Autodesk Inventor part; units mm, degrees
ref_plane "Work Plane5" through (0, 0, 76.2) normal (0, 0, 1) x (1, 0, 0)
ref_plane "Work Plane6" through (0, 0, 15.113) normal (0, 0, -1) x (-1, 0, 0)
ref_plane "Work Plane10" through (0, 0, 29.464) normal (0, 0, -1) x (-1, 0, 0)
sketch "Sketch1" plane through (0, 0, 0) normal (0, 0, 1) x (1, 0, 0)
  circle A0 centre (0, 0) radius 12.7
  circle A1 centre (0, 0) radius 6.35
  line L0 (-1.5875, 14.2875) -> (1.5875, 14.2875)
  line L1 (1.5875, 14.2875) -> (1.5875, 11.1125)
  line L2 (1.5875, 11.1125) -> (-1.5875, 11.1125)
  line L3 (-1.5875, 11.1125) -> (-1.5875, 14.2875)
  dimension "d0" = 25.4
  dimension "d4" = 12.7
  dimension "d50" = 3.175
  dimension "d51" = 3.175
  dimension "d52" = 1.5875
  dimension "d53" = 14.2875
extrude "Extrusion4" add sketch "Sketch1" along normal blind 79.375 contours A0 L3 L2 L1 | L1 L2 L3 A0
ref_plane "Work Plane5" through (0, 0, 76.2) normal (0, 0, 1) x (1, 0, 0)
sketch "Sketch6" plane through (0, 0, 76.2) normal (0, 0, 1) x (1, 0, 0)
  circle A0 centre (0, 0) radius 12.192
  circle A1 centre (0, 0) radius 12.7
  dimension "d24" = 24.384
extrude "Extrusion8" cut sketch "Sketch6" along normal blind 1.143
ref_plane "Work Plane6" through (0, 0, 15.113) normal (0, 0, -1) x (-1, 0, 0)
ref_plane "Work Plane9" through (0, 0, 43.3324) normal (0, 0, -1) x (-1, 0, 0)
ref_plane "Work Plane10" through (0, 0, 29.464) normal (0, 0, -1) x (-1, 0, 0)
extrude "Extrusion16" cut sketch "Sketch1" along normal through all contours L1 L2 L3 A0 | A0 L3 L0 L1 picked at (0.1768, 11.638)
sketch "Sketch14" plane through (0, 0, 79.375) normal (0, 0, 1) x (1, 0, 0)
  circle A0 centre (0, 0) radius 6.35
  circle A1 centre (0, 0) radius 7.9375
  dimension "d56" = 15.875
extrude "Extrusion17" cut sketch "Sketch14" against normal blind 7.9375
sketch "Sketch15" plane through (0, 0, 0) normal (0, 0, -1) x (-1, 0, 0)
  circle A0 centre (0, 0) radius 6.35
  circle A1 centre (0, 0) radius 7.9375
  dimension "d59" = 15.875
extrude "Extrusion18" cut sketch "Sketch15" against normal blind 7.9375
ref_plane "Work Plane13" through (0, 0, 6.35) normal (0, 0, -1) x (-1, 0, 0)
sketch "Sketch16" plane through (0, 0, 6.35) normal (0, 0, -1) x (-1, 0, 0)
  arc A0 (-1.5875, 12.6004) -> (1.5875, 12.6004) centre (0, 0) ccw
  line L0 (-1.5875, 12.6004) -> (-1.5875, 11.1125)
  line L1 (-1.5875, 11.1125) -> (1.5875, 11.1125)
  line L2 (1.5875, 11.1125) -> (1.5875, 12.6004)
  circle A1 centre (0, 0) radius 15.875
  circle A2 centre (0, 0) radius 14.2875
  dimension "d63" = 31.75
  dimension "d68" = 28.575
extrude "Extrusion19" add sketch "Sketch16" against normal blind 3.175 contours A1 | A2
sketch "Sketch17" plane through (0, 0, 0) normal (0, 0, -1) x (-1, 0, 0)
  line L0 (-1.5875, 11.1125) -> (-1.5875, 12.6004)
  arc A0 (-1.5875, 12.6004) -> (1.5875, 12.6004) centre (0, 0) ccw
  line L1 (1.5875, 12.6004) -> (1.5875, 11.1125)
  line L2 (1.5875, 11.1125) -> (-1.5875, 11.1125)
  arc A1 (1.5875, 12.6004) -> (-1.5875, 12.6004) centre (0, 0) ccw
extrude "Extrusion20" add sketch "Sketch17" against normal blind 6.35 contours L0 A1 L1 L2
extrude "Extrusion21" add sketch "Sketch16" against normal blind 6.35 contours A2
equation "\"d51\" = d50"
properties part number "turn shaft 3"
For this review, take the finished solid that the model builds, in its own axes (mm). A direction names the side the tool comes from. Round coordinates to 2 decimals unless told otherwise and drop trailing zeros. Use CSV: the item, a comma, the result in double quotes.
1) Clearance check with flat-ended pins moving along their axes: pin 1 Ø1.6 at (x, z) = (-1, 51.5) entering from +Y; pin 2 Ø1.2 at (y, z) = (12, 48.5) entering from +X; pin 3 Ø2 at (x, z) = (-0.5, 40.5) entering from -Y; pin 4 Ø7.5 at (x, y) = (0, 0) entering from +Z. State where each tip first meets the part, or that it passes through.
Conclusion:
pin 1,"stops at y = 12.6"
pin 2,"stops at x = 5.6"
pin 3,"stops at y = -12.7"
pin 4,"passes through"
2) The part is to be moulded in two halves that separate along Z. For faces 1 (the flat face through (7, 11, 6.35)), 2 (the cylindrical face through (0.51, -12.18, 76.76)), 3 (the cylindrical face through (-1.72, -7.75, 75.46)), say which applies: pulls with the +Z half, pulls with the -Z half, needs draft (parallel to the pull), parting line crosses it, or undercut.
Conclusion:
face 1,"pulls with the -Z half"
face 2,"undercut"
face 3,"needs draft"
3) For faces 4 (the cylindrical face through (0.54, -12.69, 44.01)), 5 (the flat face through (-12.3, -1.9, 76.2)), 6 (the flat face through (-1.588, 12, 46)), 7 (the flat face through (0, 7, 7.938)), list the 3-axis set-ups (+Z, -Z, +X, -X, +Y, -Y) from which the entire face can be reached by the end or side of a thin tool; tool diameter is ignored.
Conclusion:
face 4,"+Z"
face 5,"none"
face 6,"+Z, +Y"
face 7,"-Z"
4) Wall thickness on line 1 along Z through (x, y) = (-13.5, 8) (3 decimals); line 2 along X through (y, z) = (-3.5, 46); line 3 along Y through (x, z) = (0, 75): over which ranges is each line inside the solid? List them lowest first. Write a range as from..to.
Conclusion:
line 1,"z = 6.35..9.525"
line 2,"x = -12.21..-5.3, 5.3..12.21"
line 3,"y = -12.7..-7.94, 7.94..11.11"
